Source: three-view drawing plus pictorial views. Frame: mm from the lowest corner of the part. Round coordinates to 2 decimals unless told otherwise and drop trailing zeros. Order: outer loops, then holes, each group sorted by start corner. A loop starts at its lowest first (then second) coordinate and runs counter-clockwise, first axis right, second up. Notation, with made-up numbers: (29, -3.5) -> (52, -3.5) arc R13 cw to (52, 8.5) -> close; hole circle Ø6 at (35, 50.5). An arc over 180 degrees is marked (long way). Answer as CSV lines item,"result".
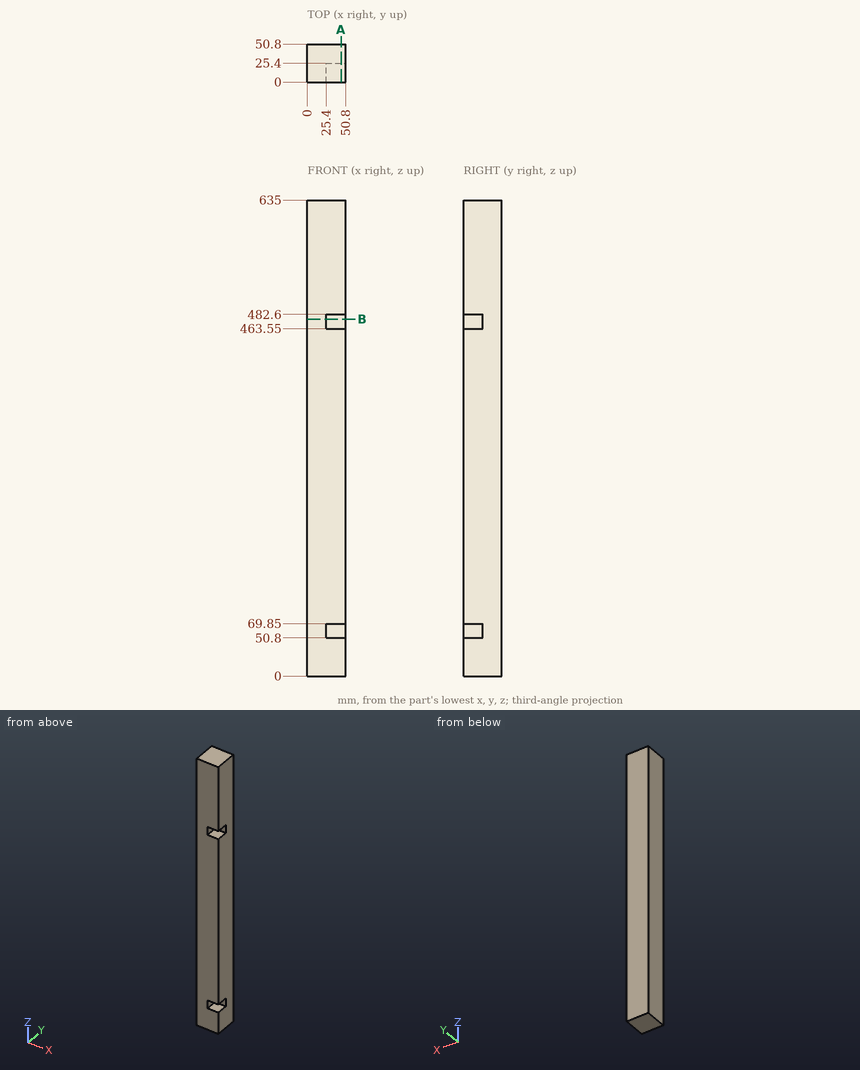
1. Pin query (flat end, axial travel): pin 1 (15 mm diameter, centred on x = 40, z = 58.5, fed in from -Y); pin 2 (9.5 mm diameter, centred on y = 6.5, z = 472.5, fed in from +X). Return the tip coordinate at first contact, or that it passes through.
Results below:
pin 1,"y = 25.4"
pin 2,"x = 25.4"
2. Section query A-A on x = 45. Return loops of the section in (y, z), and give its area (3 significant figures).
Results below:
outline,"(0, 0) -> (50.8, 0) -> (50.8, 635) -> (0, 635) -> (0, 482.6) -> (25.4, 482.6) -> (25.4, 463.55) -> (0, 463.55) -> (0, 69.85) -> (25.4, 69.85) -> (25.4, 50.8) -> (0, 50.8) -> close"
area,"31,300 mm2"
3. Section query B-B on z = 476. Return loops of the section in (x, y).
Results below:
outline,"(0, 0) -> (25.4, 0) -> (25.4, 25.4) -> (50.8, 25.4) -> (50.8, 50.8) -> (0, 50.8) -> close"
4. Line query: L1, parallel to Z at x = 43, y = 12; L2, parallel to Y at x = 45, z = 479. Output: solid intervals per line, ascending. Write a range as [from, to].
Results below:
L1,"[0, 50.8], [69.85, 463.55], [482.6, 635]"
L2,"[25.4, 50.8]"
